The figure shows three views and two pictorial views of one solid part (mm, origin at its lowest corner). Answer the questions. A direction names the side the tool comes from. Coordinates: 2 decimals unless noted, no trailing zeros. Loops run counter-clockwise (first coordinate to the right, second up) from the corner with the lowest first, then second, coordinate; pieces in that order, holes last. Notation, with made-up numbers: (-37.5, 36.5) -> (21.5, 36.5) arc R9 cw to (21.5, 43.5) -> close; hole circle Ø1 at (67, 30). An arc over 180 degrees is marked (long way). Answer as a JSON object with one key per item and string values. Group by question number.
1) Section D-D, the plane z = 4 is taken. Give the vertices of the cut face in (x, y).
2) Flat-ended cylindrical pins translate along their axes: P1, Ø1, axis at y = 8.5, z = 6.5, coming from the -X side; P2, Ø4, axis at x = 14, z = 6, coming from the +Y side; P3, Ø1.6, axis at x = 6, z = 6, coming from the -Y side. Find the tip coordinate at first contact, or state that the pin passes through.
3) Which of the six approach directions +Z, -Z, +X, -X, +Y, -Y give full straight-line access (tool end or side, diameter ignored) to the marked faces 1 and 2?
4) Consider probe 1 along X at (y, z) = (2, 6); probe 2 along Z at (x, y) = (6, 6); probe 3 along Z at (x, y) = (14.5, 5.75). Determine where each line is inside the solid, lowest interval first. Write a range as [from, to].
5) Section B-B, the plane y = 1.5 is taken. Give the vertices of the cut face in (x, z).
6) Section A-A, the plane z = 6 is taken. Give the vertices of the cut face in (x, y).
7) Determine the mould class of the marked faces 3, 4, 5 and 6 for opening direction Z: released by +Z, released by -Z, zero draft, split by the parting line, or undercut.
8) Section C-C, the plane x = 7.75 is taken. Give the vertices of the cut face in (y, z) (1 decimal), plus the area to 3 significant figures.
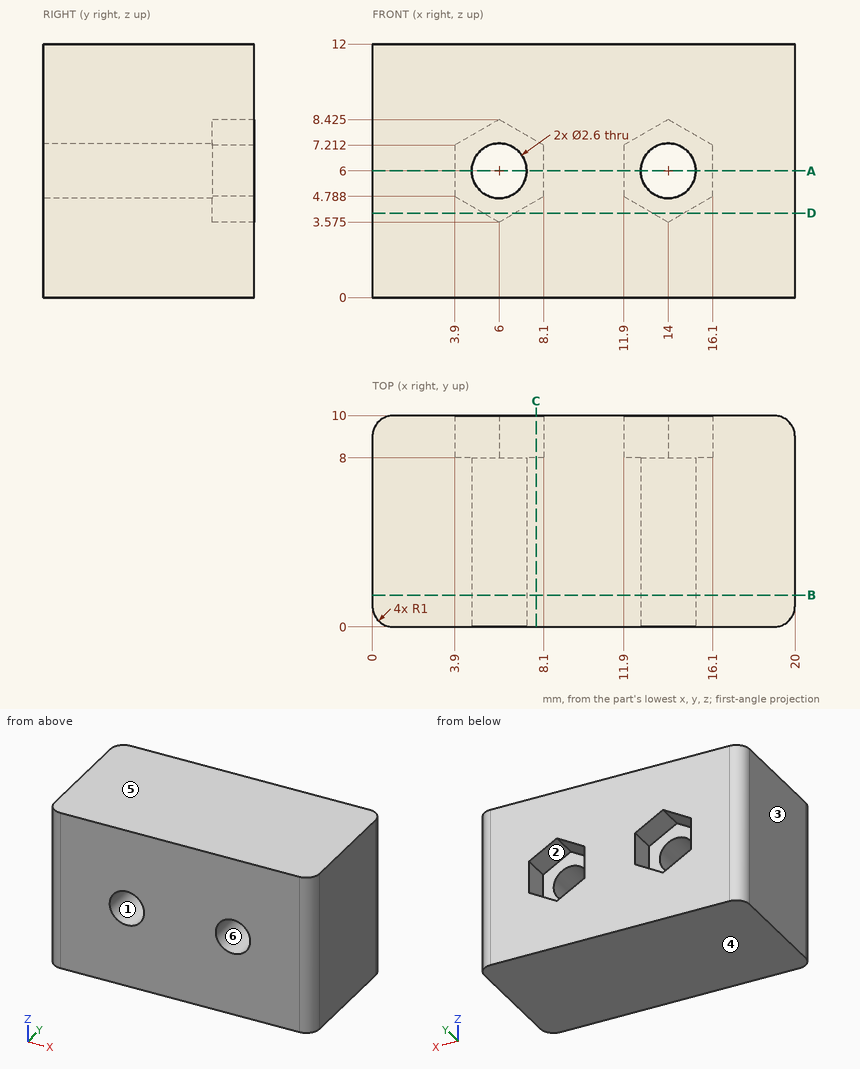
Determined:
{
 "1": {"outline": "(0, 1) arc R1 ccw to (1, 0) -> (19, 0) arc R1 ccw to (20, 1) -> (20, 9) arc R1 ccw to (19, 10) -> (14.74, 10) -> (14.74, 8) -> (13.26, 8) -> (13.26, 10) -> (6.74, 10) -> (6.74, 8) -> (5.26, 8) -> (5.26, 10) -> (1, 10) arc R1 ccw to (0, 9) -> close"},
 "2": {"P1": "x = 0", "P2": "y = 8", "P3": "through"},
 "3": {"face 1": "+Y, -Y", "face 2": "+Y"},
 "4": {"probe 1": "[0, 4.7], [7.3, 12.7], [15.3, 20]", "probe 2": "[0, 4.7], [7.3, 12]", "probe 3": "[0, 4.8], [7.2, 12]"},
 "5": {"outline": "(0, 0) -> (20, 0) -> (20, 12) -> (0, 12) -> close; hole circle Ø2.6 at (6, 6); hole circle Ø2.6 at (14, 6)"},
 "6": {"outline": "(0, 1) arc R1 ccw to (1, 0) -> (4.7, 0) -> (4.7, 8) -> (3.9, 8) -> (3.9, 10) -> (1, 10) arc R1 ccw to (0, 9) -> close; (7.3, 0) -> (12.7, 0) -> (12.7, 8) -> (11.9, 8) -> (11.9, 10) -> (8.1, 10) -> (8.1, 8) -> (7.3, 8) -> close; (15.3, 0) -> (19, 0) arc R1 ccw to (20, 1) -> (20, 9) arc R1 ccw to (19, 10) -> (16.1, 10) -> (16.1, 8) -> (15.3, 8) -> close"},
 "7": {"face 3": "zero draft", "face 4": "released by -Z", "face 5": "released by +Z", "face 6": "undercut"},
 "8": {"outline": "(0, 0) -> (10, 0) -> (10, 4.6) -> (8, 4.6) -> (8, 7.4) -> (10, 7.4) -> (10, 12) -> (0, 12) -> close", "area": "114 mm²"}
}
